Input: part model. Units: mm. Frame: model coordinates. A direction names the side the tool comes from. Coordinates: 2 decimals unless noted, no trailing zeros. Loops run counter-clockwise (first coordinate to the right, second up) from the corner with the lowest first, then second, coordinate; pieces in that order, holes last. Notation, with made-up numbers: M 60,19.25 L 76,19.25 A36 cw 76,58.25 Z; hole C 53,23.5 d2. An arc over 180 degrees is marked long. Use a Markdown table: item, result. Add a question column.
1. Section A-A on x = 0. Output: boundary loops of the cut face in (y, z) (3 decimals).
2. Line query: L1, parallel to X at y = -242, z = -11.5; L2, parallel to X at y = -328, z = -0.75; L3, parallel to Y at x = 26, z = 0.25. Output: solid intervals per line, ascending. Write a range as [from, to].
3. Section C-C on z = 8.25. Output: boundary loops of the cut face in (x, y) (3 decimals), then the cut area to 3 significant figures.
4. Set-up query: faces 5 (the flat face through (-67, -154, -12.5)), 6 (the cylindrical face through (1.004, 45.664, -0.175)). Return all of +Z, -Z, +X, -X, +Y, -Y with unobstructed straight access to the full face (end or side cutting, diameter ignored); none if empty.
5. Pin query (flat end, axial travel): pin 1 (1.5 mm diameter, centred on y = -336, z = 2, fed in from -X); pin 2 (1.5 mm diameter, centred on y = -282.5, z = -2, fed in from -X); pin 3 (5 mm diameter, centred on y = -204.5, z = -3, fed in from +X). Return the tip coordinate at first contact, or that it passes through.
6. Draft query along X for faces 1 (the flat face through (70.47, -153.62, -0.18)), 2 (the flat face through (-69.905, -149.379, -0.175)), 3 (the flat face through (-65.605, -149.379, -0.175)), 4 (the flat face through (-67, -154, 12.5)). Return one class per face: +X half, -X half, draft (parallel to the pull), parting line (faces both ways), or undercut.
7. Section B-B on y = -296. Output: boundary loops of the cut face in (x, z), then the cut area to 3 significant figures.
```python
from build123d import *

# Parameters (mm, degrees)
AUFSATZ_LINEAR_AUSTRAGEN1_DEPTH      = 12.5
AUFSATZ_LINEAR_AUSTRAGEN1_DEPTH_BACK = 12.5


with BuildPart() as part:
    # Skizze3 → Aufsatz-Linear austragen1 (new, two sides: drawn at the far end of the back side and taken through both)
    with BuildSketch(Plane.XY.offset(-AUFSATZ_LINEAR_AUSTRAGEN1_DEPTH_BACK)):
        with BuildLine():
            Line((-49.975, 0), (-90.4, -303))
            ThreePointArc((-90.4, -303), (0, -393.4), (90.4, -303))
            Line((90.4, -303), (49.975, 0))
            ThreePointArc((49.975, 0), (0, 49.975), (-49.975, 0))
        make_face()
        with BuildLine():
            Line((86.1, -303), (45.675, 0))
            ThreePointArc((45.675, 0), (0, 45.675), (-45.675, 0))
            Line((-45.675, 0), (-86.1, -303))
            ThreePointArc((-86.1, -303), (0, -389.1), (86.1, -303))
        make_face(mode=Mode.SUBTRACT)
    extrude(amount=AUFSATZ_LINEAR_AUSTRAGEN1_DEPTH + AUFSATZ_LINEAR_AUSTRAGEN1_DEPTH_BACK)


solid = part.part
```
Answers below:
| question | item | result |
|---|---|---|
| 1 | outline | M -393.4,-12.5 L -389.1,-12.5 L -389.1,12.5 L -393.4,12.5 Z; M 45.675,-12.5 L 49.975,-12.5 L 49.975,12.5 L 45.675,12.5 Z |
| 2 | L1 | x = [-82.26, -77.96], [77.96, 82.26] |
| 2 | L2 | x = [-86.87, -82.39], [82.39, 86.87] |
| 2 | L3 | y = [-389.58, -385.08], [37.55, 42.68] |
| 3 | outline | M -90.4,-303 A90.4 ccw 90.4,-303 L 49.975,0 A49.975 ccw -49.975,0 Z; hole M -86.1,-303 A86.1 ccw 86.1,-303 L 45.675,0 A45.675 ccw -45.675,0 Z |
| 3 | area | 4,440 mm² |
| 4 | face 5 | -Z, +X, -X, +Y, -Y |
| 4 | face 6 | +Z, -Z |
| 5 | pin 1 | stops at x = -84.45 |
| 5 | pin 2 | stops at x = -87.77 |
| 5 | pin 3 | stops at x = 77.59 |
| 6 | face 1 | +X half |
| 6 | face 2 | -X half |
| 6 | face 3 | undercut |
| 6 | face 4 | draft |
| 7 | outline | M -89.47,-12.5 L -85.17,-12.5 L -85.17,12.5 L -89.47,12.5 Z; M 85.17,-12.5 L 89.47,-12.5 L 89.47,12.5 L 85.17,12.5 Z |
| 7 | area | 215 mm² |
